For this review, take the finished solid that the model builds, in its own axes (mm). Face numbers are marked on the shaded views. A direction names the side the tool comes from. Coordinates: 2 decimals unless noted, no trailing zeros. Order: outer loops, then holes, each group sorted by start corner. A loop starts at its lowest first (then second) coordinate and runs counter-clockwise, first axis right, second up. Notation, with made-up numbers: M 17.25,67.5 L 66.25,67.5 A24 cw 66.25,95.5 Z; hole C -39.75,35.25 d10. An arc over 180 degrees is marked long. Use CSV: the item, a comma, the result in double quotes.
Autodesk Inventor part; units mm, degrees
ref_plane "YZ Plane" through (0, 0, 0) normal (1, 0, 0) x (0, 1, 0)
ref_plane "XZ Plane" through (0, 0, 0) normal (0, 1, 0) x (-1, 0, 0)
ref_plane "XY Plane" through (0, 0, 0) normal (0, 0, 1) x (1, 0, 0)
sketch "Esquisse1" plane through (0, 0, 0) normal (0, 1, 0) x (-1, 0, 0)
  arc A0 (-8.5, 9.1652) -> (8.5, 9.1652) centre (0, 0) ccw
  line L0 (8.5, 9.1652) -> (8.5, 14.1652)
  line L1 (-8.5, 9.1652) -> (-8.5, 14.1652)
  arc A1 (-8.5, 14.1652) -> (8.5, 14.1652) centre (0, 0) ccw
  line L2 (-12.0741, -3.2352) -> (-15.9568, -4.2756)
  line L3 (23.1276, 0) -> (-23.1276, 0)
  point P0 (-14.1537, -8.5191)
  dimension "d0" = 12.5
  dimension "d1" = 5
  dimension "d2" = 17
  dimension "d11" = 15
extrude "Extrusion1" add sketch "Esquisse1" along normal mid plane 20 contours A0 L3 A1 L2 | A0 L0 A1 L3 picked at (15.0221, -1.3088)
chamfer "Chanfrein1" distance 1 angle 45 2 edges at (-8.5, 0, 14.1652) (12.0741, 0, -3.2352)
chamfer "Chanfrein2" distance 0.5 angle 45 2 edges at (-9.5419, 10, -13.4853) (-9.5419, -10, -13.4853)
chamfer "Chanfrein3" distance 2 angle 45 1 edges at (15.9568, 0, -4.2756)
properties part number "viseur_base"
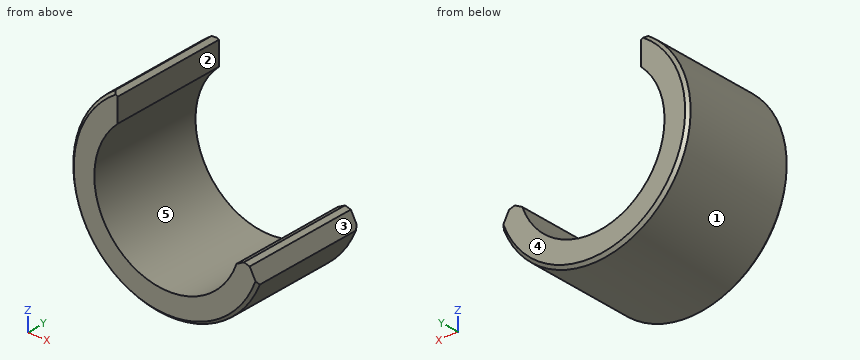
Item 1: Draft analysis for pull direction Z (two halves, no side actions). For the marked faces 3, 4 and 5, state which applies: released by +Z, released by -Z, zero draft, split by the parting line, or undercut.
Solutions:
face 3,"released by +Z"
face 4,"zero draft"
face 5,"undercut"
Item 2: Add section A-A on z = 0. State the section outline as (x, y) points.
Solutions:
outline,"M -16.52,-9.5 L -16.02,-10 L -12.5,-10 L -12.5,10 L -16.02,10 L -16.52,9.5 Z"
Item 3: To check wall thickness, follow line 1 along Z through (x, y) = (0, -3); line 2 along Z through (x, y) = (-9, 2). State the ranges of each line that lie inside material, in increasing order. Write a range as [from, to].
Solutions:
line 1,"[-16.52, -12.5]"
line 2,"[-13.85, -8.67], [8.67, 13.44]"
Item 4: For the marked faces 1 and 2, list the 3-axis set-ups (+Z, -Z, +X, -X, +Y, -Y) from which the entire face can be reached by the end or side of a thin tool; tool diameter is ignored.
Solutions:
face 1,"+Y, -Y"
face 2,"+Z, +X, +Y, -Y"
Item 5: Add section C-C on x = 0. State the section outline as (y, z) points.
Solutions:
outline,"M -10,-16.02 L -9.5,-16.52 L 9.5,-16.52 L 10,-16.02 L 10,-12.5 L -10,-12.5 Z"
Item 6: Add section B-B on y = -4.75. State the section outline as (x, z) points, and give its area (3 significant figures).
Solutions:
outline,"M -9.34,13.62 A16.52 ccw long 15.32,-6.17 L 14.02,-3.76 L 13.04,-3.49 L 11.78,-4.19 A12.5 cw long -8.5,9.17 L -8.5,13.17 Z"
area,"220 mm^2"
Item 7: Clearance check with flat-ended pins moving along their axes: pin 1 Ø1 at (y, z) = (-6.5, 4) entering from +X; pin 2 Ø4 at (x, y) = (-9.5, 6.5) entering from -Z; pin 3 Ø2 at (y, z) = (4.5, 11) entering from +X; pin 4 Ø10 at (x, z) = (-3.5, -7) entering from +Y. State where each tip first meets the part, or that it passes through.
Solutions:
pin 1,"x = -11.66"
pin 2,"z = -14.72"
pin 3,"x = -8.5"
pin 4,"y = 10"
